Could you check a few things on this model? Use its own coordinates, in mm. Face numbers are marked on the shaded views. A direction names the side the tool comes from. Coordinates: 2 decimals unless noted, no trailing zeros. Order: outer loops, then holes, each group sorted by start corner. A loop starts at its lowest first (then second) coordinate and runs counter-clockwise, first axis right, second up. Notation, with made-up numbers: (41, 67.25) - (54, 67.25) arc R17 cw to (54, 80.25) - close; hole circle Ø8 at (74.25, 53.5). An arc over 180 degrees is marked (long way). Answer as a JSON object with one key per item and string values. Group by question number.
(1) Imagine slicing it at B-B, the plane y = 14. Give the number of separate pieces and of enclosed holes in the cut face, and give its area (3 significant figures).
(2) We'd pull the mould along X, two halves only. Please class the marked faces 1, 2 and 3: pulls with the +X half, pulls with the -X half, needs draft (parallel to the pull), parting line crosses it, or undercut.
(3) Will this pin go through, and if not, where does the flat tip stop? P1, Ø1.2, axis at x = -5, z = 22.5, coming from the +Y side.
(4) Imagine slicing it at A-A, the plane x = 1.5. Write out the boundary of the cut face in (y, z), and give its area (3 significant figures).
(5) Please list where these lines run through material, in increasing order: probe 1 along X at (y, z) = (3.75, 4.5); probe 2 along X at (y, z) = (18.25, 12); probe 3 along X at (y, z) = (15.75, 22).
(6) Which directions (+Z, -Z, +X, -X, +Y, -Y) give clear straight access to the entire face, cutting with the end or side of a thin tool? Please do the marked faces 4, 5 and 6.
(7) Imagine slicing it at C-C, the plane x = -36.5. Write out the boundary of the cut face in (y, z).
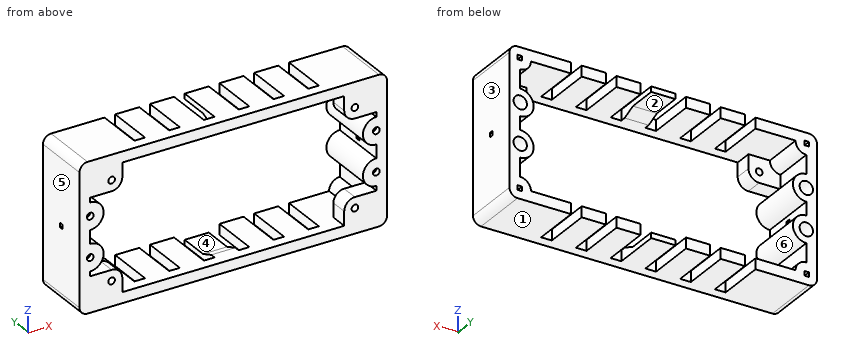
from build123d import *

# Parameters (mm, degrees)
EXTRUDE_1_DEPTH     = 22
SKETCH_4_W          = 12
SKETCH_4_H          = 6.5
EXTRUDE_3_DEPTH     = 9.25
FILLET_1_R          = 4
SKETCH_5_W          = 12
SKETCH_5_H          = 6.5
EXTRUDE_4_DEPTH     = 9.25
FILLET_2_R          = 4
SKETCH_6_R          = 2.5
CUT_EXTRUDE_1_DEPTH = 20
SKETCH_7_R          = 1.25
CUT_EXTRUDE_2_DEPTH = 20
SKETCH_8_R          = 1.25
CUT_EXTRUDE_3_DEPTH = 20
SKETCH_9_W          = 1.7
SKETCH_9_H          = 1.7
CUT_EXTRUDE_4_DEPTH = 120
EXTRUDE_5_DEPTH     = 15.5
SKETCH_11_W         = 1.7
SKETCH_11_H         = 1.7
CUT_EXTRUDE_5_DEPTH = 5
SKETCH_12_W         = 4
SKETCH_12_H         = 18
CUT_EXTRUDE_6_DEPTH = 71
SKETCH_13_W         = 9
SKETCH_13_H         = 2
CUT_EXTRUDE_7_DEPTH = 11
CHAMFER_1_SIZE      = 5
CHAMFER_1_SIZE_2    = 2.020131129


with BuildPart() as part:
    # Эскиз1 → Бобышка-Вытянуть1 (new body)
    with BuildSketch(Plane(origin=(0, 0, 0), x_dir=(1, 0, 0), z_dir=(0, 1, 0))):
        with BuildLine():
            Line((-53.32847827, 30.587656235), (55.67152173, 30.587656235))
            ThreePointArc((55.67152173, 30.587656235), (57.792842073, 29.708976578), (58.67152173, 27.587656235))
            Line((58.67152173, 27.587656235), (58.67152173, -21.412343765))
            ThreePointArc((58.67152173, -21.412343765), (57.792842073, -23.533664109), (55.67152173, -24.412343765))
            Line((55.67152173, -24.412343765), (-53.32847827, -24.412343765))
            ThreePointArc((-53.32847827, -24.412343765), (-55.449798614, -23.533664109), (-56.32847827, -21.412343765))
            Line((-56.32847827, -21.412343765), (-56.32847827, 27.587656235))
            ThreePointArc((-56.32847827, 27.587656235), (-55.449798614, 29.708976578), (-53.32847827, 30.587656235))
        make_face()
        with BuildLine():
            Line((-52.32847827, 26.587656235), (-52.32847827, 15.587656235))
            ThreePointArc((-52.32847827, 15.587656235), (-47.32847827, 10.587656235), (-52.32847827, 5.587656235))
            Line((-52.32847827, 5.587656235), (-52.32847827, 0.587656235))
            ThreePointArc((-52.32847827, 0.587656235), (-47.32847827, -4.412343765), (-52.32847827, -9.412343765))
            Line((-52.32847827, -9.412343765), (-52.32847827, -20.412343765))
            Line((-52.32847827, -20.412343765), (54.67152173, -20.412343765))
            Line((54.67152173, -20.412343765), (54.67152173, -9.412343765))
            ThreePointArc((54.67152173, -9.412343765), (49.67152173, -4.412343765), (54.67152173, 0.587656235))
            Line((54.67152173, 0.587656235), (54.67152173, 5.587656235))
            ThreePointArc((54.67152173, 5.587656235), (49.67152173, 10.587656235), (54.67152173, 15.587656235))
            Line((54.67152173, 15.587656235), (54.67152173, 26.587656235))
            Line((54.67152173, 26.587656235), (-52.32847827, 26.587656235))
        make_face(mode=Mode.SUBTRACT)
    extrude(amount=EXTRUDE_1_DEPTH)

    # Эскиз4 → Бобышка-Вытянуть3 (add)
    with BuildSketch(Plane(origin=(0, 0, 20.412343765), x_dir=(-1, 0, 0), z_dir=(0, 0, -1))):
        with Locations((46.32847827, 3.25)):
            Rectangle(SKETCH_4_W, SKETCH_4_H)
        with Locations((-48.67152173, 3.25)):
            Rectangle(SKETCH_4_W, SKETCH_4_H)
    extrude(amount=EXTRUDE_3_DEPTH)

    # Скругление1
    fillet_1_edges = [part.edges().sort_by_distance(p)[0] for p in [
        (-40.32847827, 3.25, 11.162343765),
        (42.67152173, 3.25, 11.162343765),
    ]]
    fillet(fillet_1_edges, radius=FILLET_1_R)

    # Эскиз5 → Бобышка-Вытянуть4 (add)
    with BuildSketch(Plane.XY.offset(-26.587656235)):
        with Locations((-46.32847827, 3.25)):
            Rectangle(SKETCH_5_W, SKETCH_5_H)
        with Locations((48.67152173, 3.25)):
            Rectangle(SKETCH_5_W, SKETCH_5_H)
    extrude(amount=EXTRUDE_4_DEPTH)

    # Скругление2
    fillet_2_edges = [part.edges().sort_by_distance(p)[0] for p in [
        (-40.32847827, 3.25, -17.337656235),
        (42.67152173, 3.25, -17.337656235),
    ]]
    fillet(fillet_2_edges, radius=FILLET_2_R)

    # Эскиз6 → Вырез-Вытянуть1 (cut)
    with BuildSketch(Plane(origin=(0, 22, 0), x_dir=(1, 0, 0), z_dir=(0, 1, 0))):
        with Locations(Location((-52.32847827, 10.587656235, 0), (0, 0, 270))):
            Circle(SKETCH_6_R)
        with Locations(Location((-52.32847827, -4.412343765, 0), (0, 0, 270))):
            Circle(SKETCH_6_R)
        with Locations(Location((54.67152173, 10.587656235, 0), (0, 0, 270))):
            Circle(SKETCH_6_R)
        with Locations(Location((54.67152173, -4.412343765, 0), (0, 0, 270))):
            Circle(SKETCH_6_R)
    extrude(amount=-CUT_EXTRUDE_1_DEPTH, mode=Mode.SUBTRACT)

    # Эскиз7 → Вырез-Вытянуть2 (cut)
    with BuildSketch(Plane(origin=(0, 6.5, 0), x_dir=(1, 0, 0), z_dir=(0, 1, 0))):
        with Locations(Location((-44.32847827, 21.337656235, 0), (0, 0, 270))):
            Circle(SKETCH_7_R)
        with Locations(Location((46.67152173, 21.337656235, 0), (0, 0, 270))):
            Circle(SKETCH_7_R)
        with Locations(Location((46.67152173, -15.162343765, 0), (0, 0, 270))):
            Circle(SKETCH_7_R)
        with Locations(Location((-44.32847827, -15.162343765, 0), (0, 0, 270))):
            Circle(SKETCH_7_R)
    extrude(amount=-CUT_EXTRUDE_2_DEPTH, mode=Mode.SUBTRACT)

    # Эскиз8 → Вырез-Вытянуть3 (cut)
    with BuildSketch(Plane(origin=(0, 2, 0), x_dir=(1, 0, 0), z_dir=(0, 1, 0))):
        with Locations(Location((-52.32847827, 10.587656235, 0), (0, 0, 270))):
            Circle(SKETCH_8_R)
        with Locations(Location((-52.32847827, -4.412343765, 0), (0, 0, 270))):
            Circle(SKETCH_8_R)
        with Locations(Location((54.67152173, 10.587656235, 0), (0, 0, 270))):
            Circle(SKETCH_8_R)
        with Locations(Location((54.67152173, -4.412343765, 0), (0, 0, 270))):
            Circle(SKETCH_8_R)
    extrude(amount=-CUT_EXTRUDE_3_DEPTH, mode=Mode.SUBTRACT)

    # Эскиз9 → Вырез-Вытянуть4 (cut)
    with BuildSketch(Plane.ZY.offset(56.32847827)):
        with Locations((-3.087656235, 11)):
            Rectangle(SKETCH_9_W, SKETCH_9_H)
    extrude(amount=-CUT_EXTRUDE_4_DEPTH, mode=Mode.SUBTRACT)

    # Эскиз10 → Бобышка-Вытянуть5 (add)
    with BuildSketch(Plane(origin=(0, 6.5, 0), x_dir=(1, 0, 0), z_dir=(0, 1, 0))):
        with BuildLine():
            Line((-52.32847827, 22.587656235), (-52.32847827, 26.587656235))
            Line((-52.32847827, 26.587656235), (-48.32847827, 26.587656235))
            ThreePointArc((-48.32847827, 26.587656235), (-49.500051146, 23.75922911), (-52.32847827, 22.587656235))
        make_face()
        with BuildLine():
            Line((-52.32847827, -16.412343765), (-52.32847827, -20.412343765))
            Line((-52.32847827, -20.412343765), (-48.32847827, -20.412343765))
            ThreePointArc((-48.32847827, -20.412343765), (-49.500051146, -17.58391664), (-52.32847827, -16.412343765))
        make_face()
        with BuildLine():
            Line((54.67152173, -16.412343765), (54.67152173, -20.412343765))
            Line((54.67152173, -20.412343765), (50.67152173, -20.412343765))
            ThreePointArc((50.67152173, -20.412343765), (51.843094605, -17.58391664), (54.67152173, -16.412343765))
        make_face()
        with BuildLine():
            Line((54.67152173, 22.587656235), (54.67152173, 26.587656235))
            Line((54.67152173, 26.587656235), (50.67152173, 26.587656235))
            ThreePointArc((50.67152173, 26.587656235), (51.843094605, 23.75922911), (54.67152173, 22.587656235))
        make_face()
    extrude(amount=EXTRUDE_5_DEPTH)

    # Эскиз11 → Вырез-Вытянуть5 (cut)
    with BuildSketch(Plane(origin=(0, 22, 0), x_dir=(1, 0, 0), z_dir=(0, 1, 0))):
        with Locations((-52.47847827, 26.737656235)):
            Rectangle(SKETCH_11_W, SKETCH_11_H)
        with Locations((54.82152173, 26.737656235)):
            Rectangle(SKETCH_11_W, SKETCH_11_H)
        with Locations((54.82152173, -20.562343765)):
            Rectangle(SKETCH_11_W, SKETCH_11_H)
        with Locations((-52.47847827, -20.562343765)):
            Rectangle(SKETCH_11_W, SKETCH_11_H)
    extrude(amount=-CUT_EXTRUDE_5_DEPTH, mode=Mode.SUBTRACT)

    # Эскиз12 → Вырез-Вытянуть6 (cut)
    with BuildSketch(Plane.XY.offset(24.412343765)):
        with Locations((-31.32847827, 13)):
            Rectangle(SKETCH_12_W, SKETCH_12_H)
        with Locations((-18.32847827, 13)):
            Rectangle(SKETCH_12_W, SKETCH_12_H)
        with Locations((-5.32847827, 13)):
            Rectangle(SKETCH_12_W, SKETCH_12_H)
        with Locations((7.67152173, 13)):
            Rectangle(SKETCH_12_W, SKETCH_12_H)
        with Locations((20.67152173, 13)):
            Rectangle(SKETCH_12_W, SKETCH_12_H)
        with Locations((33.67152173, 13)):
            Rectangle(SKETCH_12_W, SKETCH_12_H)
    extrude(amount=-CUT_EXTRUDE_6_DEPTH, mode=Mode.SUBTRACT)

    # Эскиз13 → Вырез-Вытянуть7 (cut)
    with BuildSketch(Plane(origin=(0, 22, 0), x_dir=(1, 0, 0), z_dir=(0, 1, 0))):
        with Locations((1.17152173, 27.587656235)):
            Rectangle(SKETCH_13_W, SKETCH_13_H)
        with Locations((1.17152173, -21.412343765)):
            Rectangle(SKETCH_13_W, SKETCH_13_H)
    extrude(amount=-CUT_EXTRUDE_7_DEPTH, mode=Mode.SUBTRACT)

    # Фаска1
    # the kernel refuses this chamfer: 5, 2.020131129 mm, written as the material it takes off along each edge
    with BuildSketch(Plane(origin=(5.67152173, 11, -26.587656235), x_dir=(0, -0.9998956380575358, 0.01444690255776391), z_dir=(-1, 0, 0))) as chamfer_1_piece_1_section:
        Polygon((CHAMFER_1_SIZE * 0.999895638058, -CHAMFER_1_SIZE * 0.0144469025578), (-CHAMFER_1_SIZE_2 * 0.014446902559, -CHAMFER_1_SIZE_2 * 0.999895638145), (0, 0), align=None)
    chamfer_1_piece_1 = extrude(amount=21.964944974, mode=Mode.PRIVATE)
    chamfer_1_piece_1 = split(chamfer_1_piece_1, bisect_by=Plane(origin=(-7.32847827, 9.333169456, -27.260900856), z_dir=(1, 0, 0)), keep=Keep.TOP, mode=Mode.PRIVATE)
    chamfer_1_piece_1 = split(chamfer_1_piece_1, bisect_by=Plane(origin=(1.17152173, 9.333169456, -28.587656235), z_dir=(0, 0, 1)), keep=Keep.TOP, mode=Mode.PRIVATE)
    add(chamfer_1_piece_1, mode=Mode.SUBTRACT)
    with BuildSketch(Plane(origin=(18.636466704, 11, 20.412343765), x_dir=(0, -0.9998956380575358, -0.01444690255776391), z_dir=(-1, 0, 0))) as chamfer_1_piece_2_section:
        Polygon((CHAMFER_1_SIZE * 0.999895638058, CHAMFER_1_SIZE * 0.0144469025578), (-CHAMFER_1_SIZE_2 * 0.014446902559, CHAMFER_1_SIZE_2 * 0.999895638145), (0, 0), align=None)
    chamfer_1_piece_2 = extrude(amount=21.964944974, mode=Mode.PRIVATE)
    chamfer_1_piece_2 = split(chamfer_1_piece_2, bisect_by=Plane(origin=(9.67152173, 9.333169456, 21.085588387), z_dir=(-1, 0, 0)), keep=Keep.TOP, mode=Mode.PRIVATE)
    chamfer_1_piece_2 = split(chamfer_1_piece_2, bisect_by=Plane(origin=(1.17152173, 9.333169456, 22.412343765), z_dir=(0, 0, -1)), keep=Keep.TOP, mode=Mode.PRIVATE)
    add(chamfer_1_piece_2, mode=Mode.SUBTRACT)


solid = part.part
Result set:
{
 "1": {"separate pieces": "12", "enclosed holes": "4", "area": "1,190 mm^2"},
 "2": {"face 1": "needs draft", "face 2": "undercut", "face 3": "pulls with the +X half"},
 "3": {"P1": "stops at y = 4"},
 "4": {"outline": "(0, -30.59) - (22, -30.59) - (22, -28.59) - (10.95, -28.59) - (6, -26.59) - (0, -26.59) - close; (0, 20.41) - (6, 20.41) - (10.95, 22.41) - (22, 22.41) - (22, 24.41) - (0, 24.41) - close", "area": "122 mm^2"},
 "5": {"probe 1": "x = -56.33 to -54.83, -49.83 to -47.33, 49.67 to 52.17, 57.17 to 58.67", "probe 2": "x = -56.33 to -52.33, 54.67 to 58.67", "probe 3": "x = -56.27 to -33.33, -29.33 to -20.33, -16.33 to -7.33, 9.67 to 18.67, 22.67 to 31.67, 35.67 to 58.61"},
 "6": {"face 4": "+Y", "face 5": "+Z, -Z, -X, +Y, -Y", "face 6": "+Y, -Y"},
 "7": {"outline": "(0, -30.59) - (22, -30.59) - (22, -26.59) - (0, -26.59) - close; (0, 20.41) - (22, 20.41) - (22, 24.41) - (0, 24.41) - close"}
}
